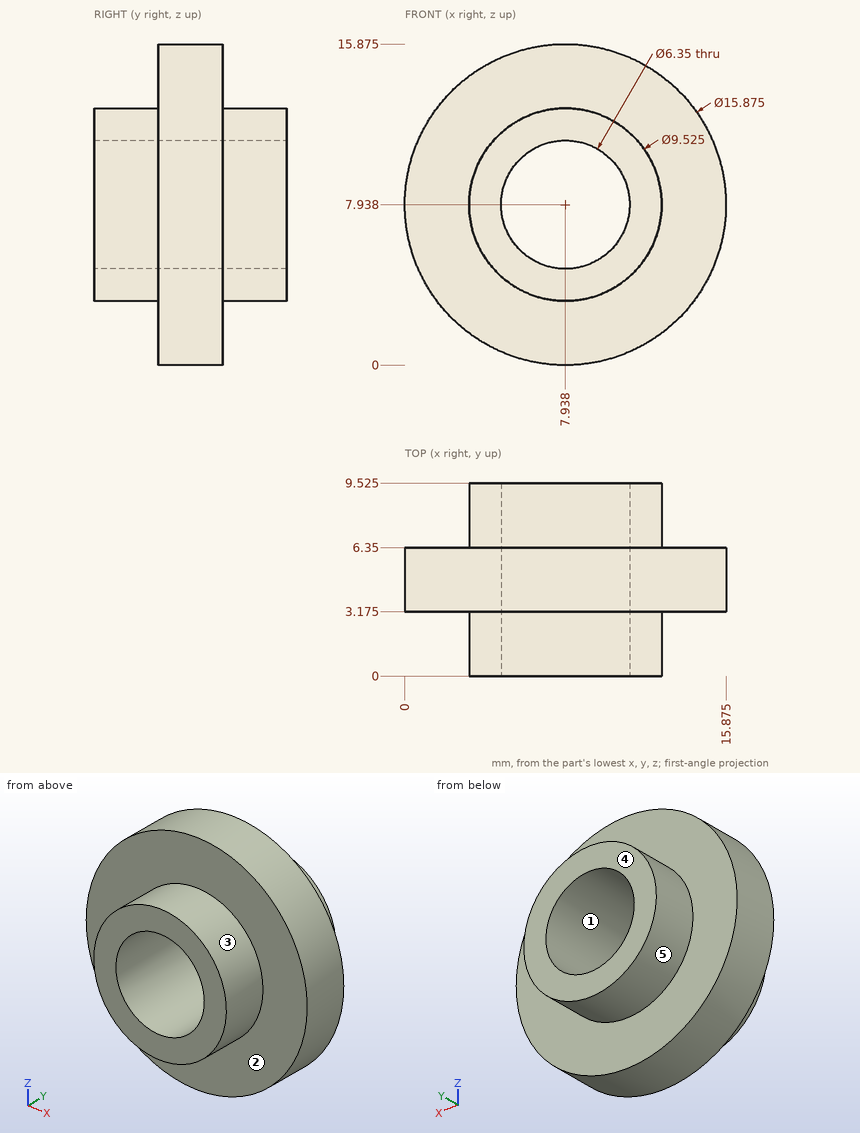
For this review, use the dimensioned drawing (mm, ordinates from the lowest corner) and the shaded views. A direction names the side the tool comes from. Coordinates: 2 decimals unless noted, no trailing zeros. Use a Markdown table: item, result. Add a question column.
1. Machinability: for the marked faces 4 and 5, which of the approach directions +Z, -Z, +X, -X, +Y, -Y give a long, thin tool a straight path to every point of the face, cutting with its end or side? Answer none if there is none.
2. Draft analysis for pull direction X (two halves, no side actions). For the marked faces 1, 2 and 3, state which applies: pulls with the +X half, pulls with the -X half, needs draft (parallel to the pull), parting line crosses it, or undercut.
3. To check wall thickness, follow line 1 (X direction, y = 7, z = 10.75) (1 decimal); line 2 (X direction, y = 8.25, z = 9.25) (1 decimal); line 3 (Z direction, x = 9.5, y = 3.5) (1 decimal). State the ranges of each line that lie inside material, in increasing order.
4. Clearance check with flat-ended pins moving along their axes: pin 1 Ø5 at (y, z) = (3.5, 11.5) entering from -X; pin 2 Ø5.5 at (x, z) = (7.94, 7.94) entering from +Y. State where each tip first meets the part, or that it passes through.
Returned:
| question | item | result |
|---|---|---|
| 1 | face 4 | +Z, -Z, +X, -X, +Y |
| 1 | face 5 | +Y |
| 2 | face 1 | undercut |
| 2 | face 2 | needs draft |
| 2 | face 3 | parting line crosses it |
| 3 | line 1 | x = 4.1 to 6.5, 9.4 to 11.8 |
| 3 | line 2 | x = 3.4 to 5, 10.8 to 12.5 |
| 3 | line 3 | z = 0.2 to 5.2, 10.7 to 15.7 |
| 4 | pin 1 | stops at x = 0.07 |
| 4 | pin 2 | passes through |
